```python
from build123d import *

# Parameters (mm, degrees)
BOSS_EXTRUDE1_DEPTH = 2.54
SKETCH3_R           = 8.128
CUT_EXTRUDE1_DEPTH  = 2.54
CUT_EXTRUDE2_DEPTH  = 3.54


with BuildPart() as part:
    # Sketch2 → Boss-Extrude1 (new body)
    with BuildSketch(Plane.XY):
        Polygon((-63.5, 2.4), (63.5, 2.4), (19.505909488, 27.8), (-63.5, 27.8), align=None)
    extrude(amount=-BOSS_EXTRUDE1_DEPTH)

    # Sketch3 → Cut-Extrude1 (cut)
    with BuildSketch(Plane.XY):
        with Locations((-50.434775134, 15.906072529)):
            Circle(SKETCH3_R)
    extrude(amount=-CUT_EXTRUDE1_DEPTH, mode=Mode.SUBTRACT)

    # Sketch4 → Cut-Extrude2 (cut, through all)
    with BuildSketch(Plane(origin=(0, 0, -2.54), x_dir=(-1, 0, 0), z_dir=(0, 0, -1))):
        Polygon((-41.105403431, 7.6), (-32.667342272, 7.6), (-32.667342272, 2.4), (-41.105403431, 2.4), (-42.967342272, 4), (-42.967342272, 6), align=None)
    extrude(amount=-CUT_EXTRUDE2_DEPTH, mode=Mode.SUBTRACT)


solid = part.part
```
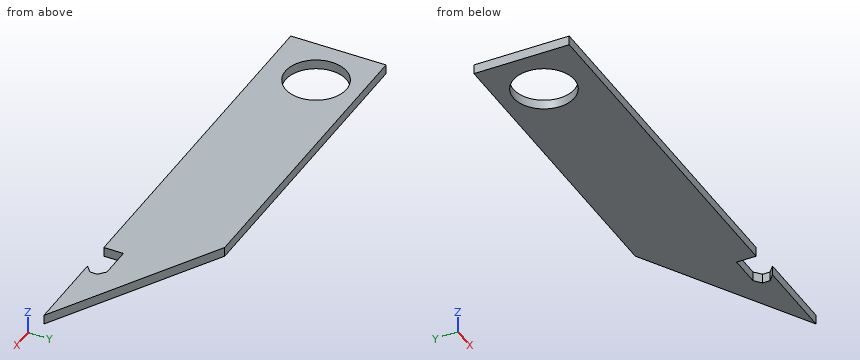
CAD build for the part. Positions are in the model's coordinates, mm. Round coordinates to 2 decimals unless told otherwise and drop trailing zeros. Order: outer loops, then holes, each group sorted by start corner. A loop starts at its lowest first (then second) coordinate and runs counter-clockwise, first axis right, second up.
Item 1: Saw through at A-A on x = -54.5. Write the cut outline in (y, z).
Item 2: Probe line 1 along X through (y, z) = (14.75, -1.15); line 2 along X through (y, z) = (19.25, -1.1); line 3 along Y through (x, z) = (30, -1.7). List the from-to ranges inside material, lowest first.
Item 3: Saw through at B-B on y = 18. Write the cut outline in (x, z), then the cut area to 3 significant figures.
Item 4: Pin check, flat tips, straight feed: pin 1 (1.3 mm diameter, centred on y = 5.5, z = -1, fed in from +X); pin 2 (1.5 mm diameter, centred on x = -41, y = 22.5, fed in from +Z); pin 3 (0.8 mm diameter, centred on x = 38.5, z = -1, fed in from -Y). Stop position of each tip, or through.
Item 5: Saw through at C-C on z = -1.8. Write the cut outline in (x, y).
Item 6: Saw through at D-D on x = 48. Write the cut outline in (y, z).
Reported:
1. outline: (2.4, -2.54) - (8.87, -2.54) - (8.87, 0) - (2.4, 0) - close; (22.94, -2.54) - (27.8, -2.54) - (27.8, 0) - (22.94, 0) - close
2. line 1: x = -63.5 to -58.48, -42.39 to 42.11
2. line 2: x = -63.5 to -57.84, -43.03 to 34.31
2. line 3: y = 2.4 to 21.74
3. outline: (-63.5, -2.54) - (-58.29, -2.54) - (-58.29, 0) - (-63.5, 0) - close; (-42.58, -2.54) - (36.48, -2.54) - (36.48, 0) - (-42.58, 0) - close
3. area: 214 mm2
4. pin 1: stops at x = 59.26
4. pin 2: stops at z = 0
4. pin 3: stops at y = 7.6
5. outline: (-63.5, 2.4) - (32.67, 2.4) - (32.67, 7.6) - (41.11, 7.6) - (42.97, 6) - (42.97, 4) - (41.11, 2.4) - (63.5, 2.4) - (19.51, 27.8) - (-63.5, 27.8) - close; hole circle Ø16.26 at (-50.43, 15.91)
6. outline: (2.4, -2.54) - (11.35, -2.54) - (11.35, 0) - (2.4, 0) - close
